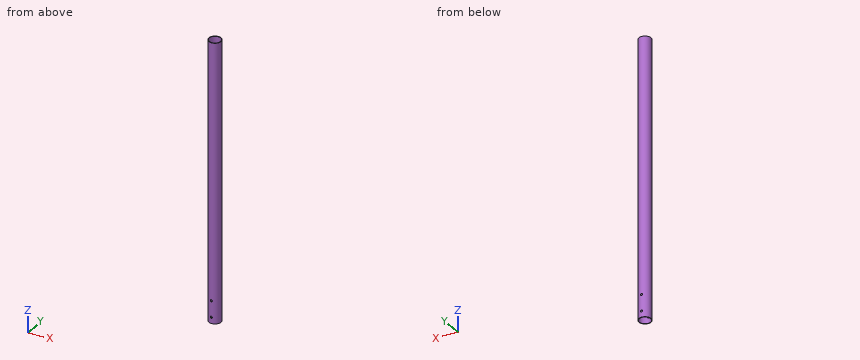
from build123d import *

# Parameters (mm, degrees)
CROQUIS1_R                 = 19.05
CROQUIS1_R_2               = 17.4625
SALIENTE_EXTRUIR1_DEPTH    = 863.6
CORTAR_EXTRUIR1_DEPTH      = 865.0201184
CORTAR_EXTRUIR1_DEPTH_BACK = 865.0201184
CROQUIS2_R                 = 3.2639


with BuildPart() as part:
    # Croquis1 → Saliente-Extruir1 (new body)
    with BuildSketch(Plane.XY):
        Circle(CROQUIS1_R)
        Circle(CROQUIS1_R_2, mode=Mode.SUBTRACT)
    extrude(amount=SALIENTE_EXTRUIR1_DEPTH)

    # Croquis2 → Cortar-Extruir1 (cut, two sides: drawn at the far end of the back side and taken through both)
    with BuildSketch(Plane(origin=(0, 0, 0), x_dir=(1, 0, 0), z_dir=(0, 1, 0)).offset(-CORTAR_EXTRUIR1_DEPTH_BACK)):
        with Locations(Location((0, -19.05, 0), (0, 0, 270))):
            Circle(CROQUIS2_R)
        with Locations(Location((0, -69.85, 0), (0, 0, 270))):
            Circle(CROQUIS2_R)
    extrude(amount=CORTAR_EXTRUIR1_DEPTH + CORTAR_EXTRUIR1_DEPTH_BACK, mode=Mode.SUBTRACT)


solid = part.part
Check sheet for the modelled part. Datum: model origin and axes. Units: mm. Give positions to 0.01 mm unless a question says otherwise; leave off trailing zeros. Write each loop counter-clockwise with the first axis right and the second up, starting at its lowest first coordinate (ties: lowest second). Pieces come first, ordered by that corner, then holes. Notation, with made-up numbers: M 59,65.25 L 108,65.25 A15 cw 108,87.25 Z; hole C 89,-6 d9. An arc over 180 degrees is marked long. Use one line per item in the form item = value.
(1) Depth check by flat-ended pin: P1, Ø4, axis at x = 5.5, z = 372.5, coming from the -Y side; P2, Ø5, axis at x = 3.5, z = 570, coming from the +Y side; P3, Ø4, axis at x = 0, z = 69.85, coming from the +Y side; P4, Ø10, axis at y = -6, z = 421.5, coming from the -X side. Enter the tip coordinate at first touch or a pass-through.
Answer block:
P1 = -18.73
P2 = 19.02
P3 = through
P4 = -19.02
(2) Section check B-B on x = -9. Record the boundary of the cut face in (y, z), plus the area to 3 significant figures.
Answer block:
outline = M -16.79,0 L -14.96,0 L -14.96,863.6 L -16.79,863.6 Z; M 14.96,0 L 16.79,0 L 16.79,863.6 L 14.96,863.6 Z
area = 3,150 mm2
(3) Material ranges on line 1 along Z through (x, y) = (0, -17.85); line 2 along Y through (x, z) = (0, 280); line 3 along X through (y, z) = (14.5, 633), recorded low to high.
Answer block:
line_1 = 0 to 15.79, 22.31 to 66.59, 73.11 to 863.6
line_2 = -19.05 to -17.46, 17.46 to 19.05
line_3 = -12.36 to -9.73, 9.73 to 12.36
(4) Section check A-A on y = 0. Record the boundary of the cut face in (x, z).
Answer block:
outline = M -19.05,0 L -17.46,0 L -17.46,863.6 L -19.05,863.6 Z; M 17.46,0 L 19.05,0 L 19.05,863.6 L 17.46,863.6 Z
